```python
from build123d import *

# Parameters (mm, degrees)
SKETCH1_R            = 60.7
BOSS_EXTRUDE1_DEPTH  = 1.5
M6_CLEARANCE_HOLE1_D = 7
CIRPATTERN1_COUNT    = 4
M2_CLEARANCE_HOLE1_D = 2.6
M3_CLEARANCE_HOLE2_D = 3.6


with BuildPart() as part:
    # Sketch1 → Boss-Extrude1 (new body)
    with BuildSketch(Plane(origin=(0, 0, 0), x_dir=(1, 0, 0), z_dir=(0, 1, 0))):
        with Locations(Location((0, 0, 0), (0, 0, 270))):
            Circle(SKETCH1_R)
    extrude(amount=BOSS_EXTRUDE1_DEPTH)

    # M6 Clearance Hole1 (through all)
    with Locations(Plane(origin=(0, 1.5, 0), x_dir=(1, 0, 0), z_dir=(0, 1, 0))):
        with Locations((-35.850313806, -35.850313806)):
            m6_clearance_hole1 = Hole(M6_CLEARANCE_HOLE1_D / 2)

    # CirPattern1: M6 Clearance Hole1 ×4 about axis
    cirpattern1_axis = Axis((0, 0, 0), (0, 1, 0))
    for i in range(1, CIRPATTERN1_COUNT):
        add(m6_clearance_hole1.rotate(cirpattern1_axis, i * 360 / CIRPATTERN1_COUNT), mode=Mode.SUBTRACT)

    # M2 Clearance Hole1 (through all)
    with Locations(Plane(origin=(0, 1.5, 0), x_dir=(1, 0, 0), z_dir=(0, 1, 0))):
        with Locations((-0.709999951, 35.730000111), (19.610000128, 35.730000136), (-5.154, -20.350313806), (-5.154, -35.350313806)):
            Hole(M2_CLEARANCE_HOLE1_D / 2)

    # M3 Clearance Hole2 (through all)
    with Locations(Plane(origin=(0, 1.5, 0), x_dir=(1, 0, 0), z_dir=(0, 1, 0))):
        with Locations((-53.86454119, 15.511690642), (-53.864546519, -14.968309358), (-32.604546519, -14.968313075), (-33.36654119, 15.511687058)):
            Hole(M3_CLEARANCE_HOLE2_D / 2)


solid = part.part
```
The model under review builds one solid part; all positions refer to its coordinate system, in mm. Coordinates: 2 decimals unless noted, no trailing zeros. Order: outer loops, then holes, each group sorted by start corner. A loop starts at its lowest first (then second) coordinate and runs counter-clockwise, first axis right, second up. Notation, with made-up numbers: (-36, -1) -> (22, -1) arc R30 ccw to (22, 33) -> close; hole circle Ø5 at (29, -17.75). An arc over 180 degrees is marked (long way). Answer in a Markdown table with one row per item. Add a question column.
Item 1: We need section A-A on y = 0.45. Give the number of separate pieces and of enclosed holes in the cut face, plus the area to 3 significant figures.
Item 2: Mouldability with a two-part tool opening along X and no side actions: class faces 1 (the cylindrical face through (60.183, 0.74, -7.902)), 2 (the cylindrical face through (-4.87, 0.74, 21.62)), 3 (the flat face through (1, 0, -1)) as +X half, -X half, draft (parallel to the pull), parting line (faces both ways), or undercut.
Item 3: We need section B-B on z = 11.5. Write out the cut boundary in (x, y), plus the area to 3 significant figures.
Item 4: To check wall thickness, follow probe 1 along Z at (x, y) = (-4.5, 0.65); probe 2 along Z at (x, y) = (-53, 0.5); probe 3 along X at (y, z) = (0.25, 16). State the ranges of each line that lie inside material, in increasing order.
Item 5: We need section C-C on x = -41.5. Write out the cut boundary in (y, z), plus the area to 3 significant figures.
Final values:
| question | item | result |
|---|---|---|
| 1 | separate pieces | 1 |
| 1 | enclosed holes | 12 |
| 1 | area | 11,400 mm2 |
| 2 | face 1 | parting line |
| 2 | face 2 | undercut |
| 2 | face 3 | draft |
| 3 | outline | (-59.6, 0) -> (59.6, 0) -> (59.6, 1.5) -> (-59.6, 1.5) -> close |
| 3 | area | 179 mm2 |
| 4 | probe 1 | z = -60.53 to 19.23, 21.47 to 34.23, 36.47 to 60.53 |
| 4 | probe 2 | z = -29.59 to -17.09, -13.93 to 13.39, 16.55 to 29.59 |
| 4 | probe 3 | x = -58.55 to -55.34, -52.39 to -34.08, -31.13 to 58.55 |
| 5 | outline | (0, -44.3) -> (1.5, -44.3) -> (1.5, 44.3) -> (0, 44.3) -> close |
| 5 | area | 133 mm2 |
